from build123d import *

# Parameters (mm, degrees)
BASPROSKE_W              = 20
BASPROSKE_H              = 11
TOOTHCUT_DEPTH           = 26.337718919
TEETHCUTS_COUNT          = 20
TEETHCUTS_ANGLE          = 342
SKETCH_2_R               = 8.5
EXTRUDE_1_DEPTH          = 12
BORSKE_R                 = 4
BORE_DEPTH               = 50.0000508
CHAMFER_1_SIZE           = 0.5
SKETCH_3_R               = 1.65
CUT_EXTRUDE_1_DEPTH      = 10
PATTERN_CIRCULAR_1_COUNT = 2
PATTERN_CIRCULAR_1_ANGLE = 90


with BuildPart() as part:
    # BasProSke → Base-Revolve (revolve)
    with BuildSketch(Plane(origin=(0, 0, 0), x_dir=(1, 0, 0), z_dir=(0, 1, 0)), mode=Mode.PRIVATE) as base_revolve_sk:
        with Locations((10, 5.5)):
            Rectangle(BASPROSKE_W, BASPROSKE_H)
    revolve(base_revolve_sk.sketch.rotate(Axis((-10, 0, 0), (1, 0, 0)), 180), axis=Axis((-10, 0, 0), (1, 0, 0)))

    # TooCutSke → ToothCut (cut, through all)
    with BuildSketch(Plane(origin=(0, 0, 0), x_dir=(0, 0, -1), z_dir=(1, 0, 0))):
        with BuildLine():
            ThreePointArc((0.499924007, 8.734705318), (0, 8.749), (-0.499924007, 8.734705318))
            ThreePointArc((-0.499924007, 8.734705318), (-0.824302243, 9.905497836), (-1.485192705, 10.924909509))
            ThreePointArc((-1.485192705, 10.924909509), (0, 11.0254), (1.485192705, 10.924909509))
            ThreePointArc((1.485192705, 10.924909509), (0.824302243, 9.905497836), (0.499924007, 8.734705318))
        make_face()
    toothcut = extrude(amount=TOOTHCUT_DEPTH, mode=Mode.SUBTRACT)

    # TeethCuts: ToothCut ×20 about axis
    teethcuts_axis = Axis((-10, 0, 0), (1, 0, 0))
    for i in range(1, TEETHCUTS_COUNT):
        add(toothcut.rotate(teethcuts_axis, i * TEETHCUTS_ANGLE / (TEETHCUTS_COUNT - 1)), mode=Mode.SUBTRACT)

    # 草圖2 → 填料-伸長1 (add)
    with BuildSketch(Plane(origin=(20, 0, 0), x_dir=(0, 0, -1), z_dir=(1, 0, 0))):
        with Locations(Location((0, 0, 0), (0, 0, 180))):
            Circle(SKETCH_2_R)
    extrude(amount=EXTRUDE_1_DEPTH)

    # BorSke → Bore (cut, symmetric)
    with BuildSketch(Plane(origin=(0, 0, 0), x_dir=(0, 0, -1), z_dir=(1, 0, 0))):
        Circle(BORSKE_R)
    extrude(amount=BORE_DEPTH, both=True, mode=Mode.SUBTRACT)

    # 導角1
    chamfer_1_edges = [part.edges().sort_by_distance(p)[0] for p in [
        (32, 0, -8.5),
    ]]
    chamfer(chamfer_1_edges, length=CHAMFER_1_SIZE)

    # 草圖3 → 除料-伸長1 (cut)
    with BuildSketch(Plane(origin=(0, 0, 0), x_dir=(1, 0, 0), z_dir=(0, 1, 0))):
        with Locations(Location((26, -0.356131442, 0), (0, 0, 270))):
            Circle(SKETCH_3_R)
    cut_extrude_1 = extrude(amount=-CUT_EXTRUDE_1_DEPTH, mode=Mode.SUBTRACT)

    # 環狀複製排列1: 除料-伸長1 ×2 about axis
    pattern_circular_1_axis = Axis((32, 0, 0), (-1, 0, 0))
    for i in range(1, PATTERN_CIRCULAR_1_COUNT):
        add(cut_extrude_1.rotate(pattern_circular_1_axis, i * PATTERN_CIRCULAR_1_ANGLE / (PATTERN_CIRCULAR_1_COUNT - 1)), mode=Mode.SUBTRACT)


solid = part.part
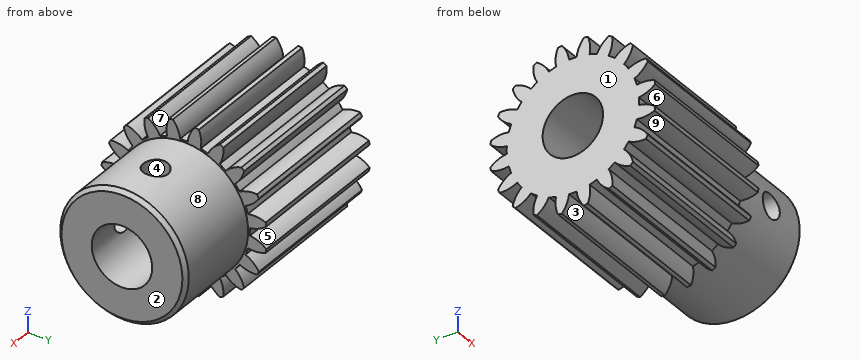
Can you work these out from the model? Positions are in its coordinate system, mm. Face numbers are marked on the shaded views. A direction names the side the tool comes from. Give positions to 0.01 mm unless a question says otherwise; leave off trailing zeros. Loops run counter-clockwise (first coordinate to the right, second up) from the corner with the lowest first, then second, coordinate; pieces in that order, holes last. Notation, with made-up numbers: (41.5, -14.5) - (46.5, -14.5) arc R25 cw to (46.5, 23.5) - close; hole circle Ø5 at (70, -16.5). An arc over 180 degrees is marked (long way). One line per item, written item: value.
(1) I'm going to push flat-ended pins straight in: pin 1 (2 mm diameter, centred on x = 26, y = 0.36, fed in from -Z); pin 2 (8 mm diameter, centred on x = 19.5, z = -3, fed in from -Y); pin 3 (5 mm diameter, centred on x = 22, z = -4.5, fed in from +Y); pin 4 (3 mm diameter, centred on x = 26, z = 0.36, fed in from -Y). Where does each tip first touch, or does it pass through?
Verdict:
pin 1: z = -8.5
pin 2: y = -10.9
pin 3: y = 9.92
pin 4: y = 3.54
(2) If we mould it in two halves opening along X, with no side actions, what happens to the marked faces 1, 2, 3 and 4? For each: released by +X, released by -X, zero draft, split by the parting line, or undercut.
Verdict:
face 1: released by -X
face 2: released by +X
face 3: zero draft
face 4: undercut
(3) If we section it at B-B, the plane z = 0: List the corners of the cut face in (x, y) for me.
Verdict:
outline: (0, -8.75) - (20, -8.75) - (20, -8.5) - (24.39, -8.5) - (24.39, -4) - (0, -4) - close; (0, 4) - (32, 4) - (32, 8) - (31.5, 8.5) - (20, 8.5) - (20, 8.75) - (0, 8.75) - close; (27.61, -8.5) - (31.5, -8.5) - (32, -8) - (32, -4) - (27.61, -4) - close
(4) If we section it at A-A, the plane x = 26: List the corners of the cut face in (y, z) for me.
Verdict:
outline: (-8.4, -1.29) arc R8.5 ccw (long way) to (2.01, 8.26) - (2.01, 3.46) arc R4 cw (long way) to (-3.78, -1.29) - close; (-8.26, 2.01) - (-3.46, 2.01) arc R4 cw to (-1.29, 3.78) - (-1.29, 8.4) arc R8.5 ccw to start
(5) I need wall thicknesses on line 1 along Y through (x, z) = (26.5, 0); line 2 along Y through (x, z) = (11, -9.5); line 3 along Y through (x, z) = (7, 0). Which ranges of each line are inside material? Lowest first, please.
Verdict:
line 1: 4 to 8.5
line 2: -5.24 to -4.19, -2.29 to -0.67, 0.67 to 2.29, 4.19 to 5.24
line 3: -8.75 to -4, 4 to 8.75
(6) If we section it at C-C, the plane y = 0: List the corners of the cut face in (x, z) for me.
Verdict:
outline: (0, -8.75) - (20, -8.75) - (20, -8.5) - (31.5, -8.5) - (32, -8) - (32, -4) - (0, -4) - close; (0, 4) - (24.39, 4) - (24.39, 8.5) - (20, 8.5) - (20, 8.75) - (0, 8.75) - close; (27.61, 4) - (32, 4) - (32, 8) - (31.5, 8.5) - (27.61, 8.5) - close
(7) On a 3-axis mill with a long thin cutter (end or side, diameter ignored), from which of +Z, -Z, +X, -X, +Y, -Y can I reach the whole of each face in a straight line? I mean the marked faces 5, 6, 7, 8 and 9. Say none if no direction works.
Verdict:
face 5: +X, -X, +Y
face 6: +X, -X, -Y
face 7: +Z, +X, -X
face 8: +X
face 9: +X, -X
